Job drawing, mm, ordinate dimensions from the low corner. One solid piece. Coordinates: 2 decimals unless noted, no trailing zeros. Order: outer loops, then holes, each group sorted by start corner. A loop starts at its lowest first (then second) coordinate and runs counter-clockwise, first axis right, second up. Notation, with made-up numbers: (-21, 38.5) -> (-5, 38.5) arc R25 cw to (-5, 73.5) -> close; hole circle Ø2 at (-4.5, -35.5). An arc over 180 degrees is marked (long way). Use CSV: the item, a comma, the result in double quotes. Start each with the question number.
(1) Cut at C-C on y = 0.75. Write the cut outline in (x, z) (1 decimal).
(2) Cut at D-D on z = 6.75. Write the cut outline in (x, y), plus the area to 3 significant figures.
(3) Pull direction X, two halves, no side cores. Call the marked faces 1, 2 and 3: pulls with the +X half, pulls with the -X half, needs draft (parallel to the pull), parting line crosses it, or undercut.
(4) Cut at B-B on x = 2.75. Write the cut outline in (y, z) (1 decimal).
(5) Cut at A-A on z = 4.5. Write the cut outline in (x, y) (1 decimal).
(6) Probe L1, parallel to X at y = 3.2, z = 4; L2, parallel to Z at x = 5.5, y = 0.25 (1 decimal); L3, parallel to X at y = 0.4, z = 2.25 (1 decimal). List the from-to ranges inside material, lowest first.
(7) Pin check, flat tips, straight feed: pin 1 Ø1.5 at (y, z) = (2.5, 1.5) entering from -X; pin 2 Ø1 at (x, z) = (3, 2) entering from -Y; pin 3 Ø4.5 at (x, z) = (3.97, 3.97) entering from +Y; pin 4 Ø1.5 at (y, z) = (1, 7) entering from +X (1 decimal). Stop position of each tip, or through.
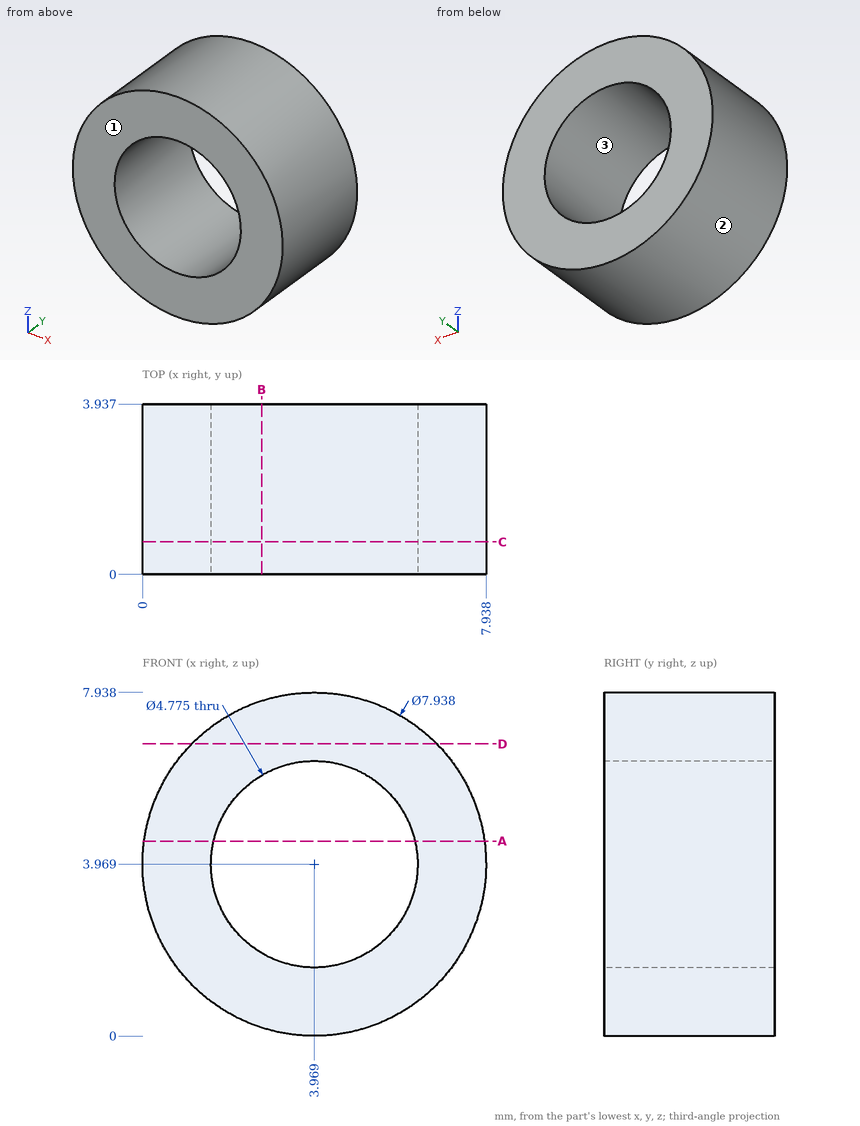
Outcome:
1,outline,"circle Ø7.9 at (4, 4); hole circle Ø4.8 at (4, 4)"
2,outline,"(1.14, 0) -> (6.8, 0) -> (6.8, 3.94) -> (1.14, 3.94) -> close"
2,area,"22.3 mm2"
3,face 1,"needs draft"
3,face 2,"parting line crosses it"
3,face 3,"undercut"
4,outline,"(0, 0.2) -> (3.9, 0.2) -> (3.9, 1.9) -> (0, 1.9) -> close; (0, 6) -> (3.9, 6) -> (3.9, 7.7) -> (0, 7.7) -> close"
5,outline,"(0, 0) -> (1.6, 0) -> (1.6, 3.9) -> (0, 3.9) -> close; (6.3, 0) -> (7.9, 0) -> (7.9, 3.9) -> (6.3, 3.9) -> close"
6,L1,"0 to 1.58, 6.36 to 7.94"
6,L2,"0.3 to 2.1, 5.8 to 7.6"
6,L3,"0.4 to 2.3, 5.6 to 7.5"
7,pin 1,"x = 0.39"
7,pin 2,"y = 0"
7,pin 3,"through"
7,pin 4,"x = 7.2"
